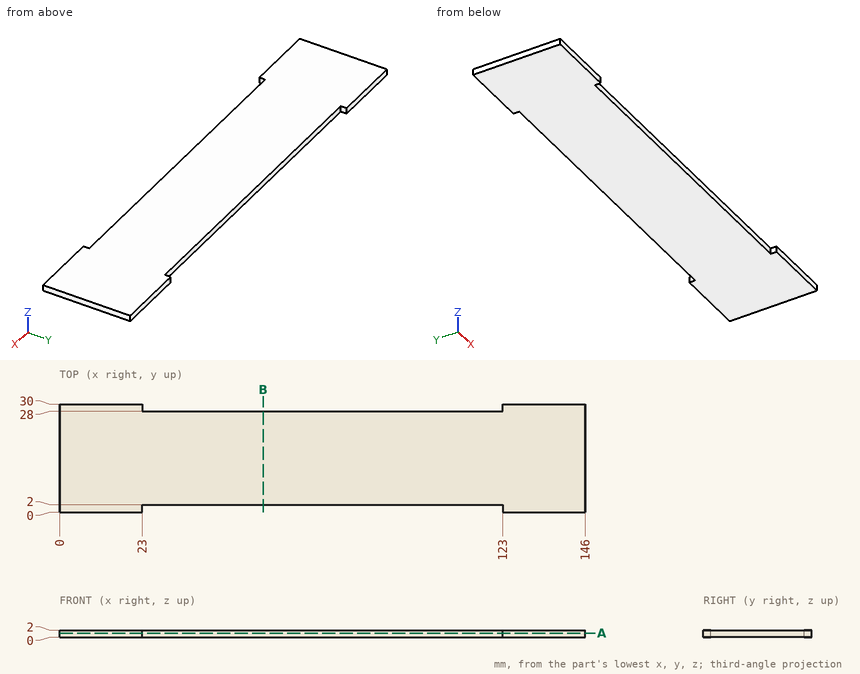
The drawing under review shows one solid part. Ordinate dimensions are in mm from its lowest x, y, z. Round coordinates to 2 decimals unless told otherwise and drop trailing zeros. Loops run counter-clockwise (first coordinate to the right, second up) from the corner with the lowest first, then second, coordinate; pieces in that order, holes last. Notation, with made-up numbers: (-6, 39.25) -> (7, 39.25) arc R17 cw to (7, 69.25) -> close; hole circle Ø3 at (-5, 5.5). An arc over 180 degrees is marked (long way). Answer in a Markdown table with one row per item.
1) Consider section B-B, the plane x = 56.5. Write out the cut boundary in (y, z), plus the area to 3 significant figures.
Taken from the geometry:
| item | result |
|---|---|
| outline | (2, 0) -> (28, 0) -> (28, 2) -> (2, 2) -> close |
| area | 52.0 mm² |
2) Consider section A-A, the plane z = 1.15. Write out the cut boundary in (x, y), plus the area to 3 significant figures.
Taken from the geometry:
| item | result |
|---|---|
| outline | (0, 0) -> (23, 0) -> (23, 2) -> (123, 2) -> (123, 0) -> (146, 0) -> (146, 30) -> (123, 30) -> (123, 28) -> (23, 28) -> (23, 30) -> (0, 30) -> close |
| area | 3,980 mm² |
3) Wall thickness on line 1 along Y through (x, z) = (67.5, 0.3): over which ranges is the line inside the solid? List them lowest first.
Taken from the geometry:
| item | result |
|---|---|
| line 1 | y = 2 to 28 |
